Design review of the part built by this model. Coordinates are the model's own, in mm. A direction names the side the tool comes from. Coordinates: 2 decimals unless noted, no trailing zeros. Loops run counter-clockwise (first coordinate to the right, second up) from the corner with the lowest first, then second, coordinate; pieces in that order, holes last. Notation, with made-up numbers: (57.25, 68) -> (107.25, 68) arc R31 cw to (107.25, 100) -> close; hole circle Ø3 at (84.5, -39.5). An arc over 180 degrees is marked (long way). Answer in a Markdown table with one row per item.
Autodesk Fusion 360 part; units mm, degrees
sketch "Sketch1" plane through (0, 0, 0) normal (0, 0, 1) x (1, 0, 0)
  line L0 (0, 0) -> (50, 0)
  line L1 (50, 0) -> (50, 56)
  line L2 (50, 56) -> (0, 56)
  line L3 (0, 56) -> (0, 0)
  dimension "d1" = 50
  dimension "d2" = 56
extrude "Extrude1" add sketch "Sketch1" along normal blind 10
sketch "Sketch2" plane through (0, 0, 10) normal (0, 0, 1) x (-1, 0, 0)
  line L0 (0, -56) -> (0, 0)
  line L1 (0, 0) -> (-50, 0)
  line L2 (-50, 0) -> (-50, -56)
  line L3 (-50, -56) -> (0, -56)
  line L4 (0, 0) -> (-6, 0)
  line L5 (-6, 0) -> (-6, -6)
  circle A0 centre (-6, -6) radius 6
  line L6 (-50, 0) -> (-44, 0)
  line L7 (-44, 0) -> (-44, -6)
  circle A1 centre (-44, -6) radius 6
  dimension "d5" = 6
  dimension "d6" = 6
  dimension "d7" = 12
  dimension "d8" = 6
  dimension "d9" = 6
  dimension "d10" = 12
extrude "Extrude2" add sketch "Sketch2" along normal blind 2 contours A0 | A1
sketch "Sketch3" plane through (0, 0, 12) normal (0, 0, 1) x (-1, 0, 0)
  circle A0 centre (-6, -6) radius 6
  line L0 (-6, -6) -> (-12, -6)
sketch "Sketch4" plane through (0, 0, 12) normal (0, 0, 1) x (-1, 0, 0)
  circle A0 centre (-44, -6) radius 6
  line L0 (-44, -6) -> (-50, -6)
hole "Hole1" at (6, 6, 12) at (44, 6, 12) direction (0, 0, -1) diameter 5.035 depth 15 tip angle 118
sketch "Sketch5" plane through (0, 56, 0) normal (0, 1, 0) x (-1, 0, 0)
  line L0 (-50, 0) -> (0, 0)
  line L1 (0, 0) -> (0, 10)
  line L2 (0, 10) -> (-50, 10)
  line L3 (-50, 10) -> (-50, 0)
  line L4 (-50, 5) -> (-45, 5)
  line L5 (0, 5) -> (-5, 5)
  dimension "d23" = 5
  dimension "d24" = 5
hole "Hole3" at (45, 56, 5) at (5, 56, 5) direction (0, -1, 0) diameter 5.035 depth 18 tip angle 118
sketch "Sketch6" plane through (0, 56, 0) normal (0, 1, 0) x (-1, 0, 0)
  circle A0 centre (-45, 5) radius 2.5175
  circle A1 centre (-5, 5) radius 2.5175
  line L0 (-50, 0) -> (0, 0)
  line L1 (0, 0) -> (0, 10)
  line L2 (0, 10) -> (-50, 10)
  line L3 (-50, 10) -> (-50, 0)
  line L4 (-45, 5) -> (-35, 5)
  line L5 (-5, 5) -> (-15, 5)
  line L6 (-35, 5) -> (-35, 0)
  line L7 (-15, 5) -> (-15, 0)
  line L8 (-35, 0) -> (-38, 0)
  line L9 (-38, 0) -> (-38, 10)
  line L10 (-38, 10) -> (-35, 10)
  line L11 (-35, 10) -> (-35, 0)
  line L12 (-15, 0) -> (-12, 0)
  line L13 (-12, 0) -> (-12, 10)
  line L14 (-12, 10) -> (-15, 10)
  line L15 (-15, 10) -> (-15, 0)
  dimension "d28" = 10
  dimension "d29" = 10
  dimension "d30" = 3
  dimension "d31" = 3
extrude "Extrude3" add sketch "Sketch6" along normal blind 2 contours L2 L4 L9 L10 L11 | L0 L4 L6 L8 L9 L11 | L0 L5 L7 L12 L13 L15 | L2 L5 L13 L14 L15
sketch "Sketch7" plane through (0, 58, 0) normal (0, 1, 0) x (-1, 0, 0)
  line L0 (-35, 10) -> (-38, 10)
  line L1 (-38, 10) -> (-38, 0)
  line L2 (-38, 0) -> (-35, 0)
  line L3 (-35, 0) -> (-35, 10)
  line L4 (-35, 0) -> (-50, 0)
  line L5 (-50, 0) -> (-50, 10)
  line L6 (-50, 10) -> (-35, 10)
  line L7 (-35, 10) -> (-35, 0)
  line L8 (-35, 0) -> (0, 0)
  line L9 (0, 0) -> (0, 10)
  line L10 (0, 10) -> (-35, 10)
  line L11 (-35, 10) -> (-35, 0)
  dimension "d34" = 15
  dimension "d35" = 10
  dimension "d36" = 35
  dimension "d37" = 10
extrude "Extrude4" add sketch "Sketch7" along normal blind 8
sketch "Sketch8" plane through (0, 66, 0) normal (0, 1, 0) x (-1, 0, 0)
  line L0 (-50, 0) -> (0, 0)
  line L1 (0, 0) -> (0, 10)
  line L2 (0, 10) -> (-50, 10)
  line L3 (-50, 10) -> (-50, 0)
  line L4 (-50, 5) -> (-45, 5)
  line L5 (0, 5) -> (-5, 5)
  dimension "d40" = 5
  dimension "d41" = 5
hole "Hole4" at (45, 66, 5) at (5, 66, 5) direction (0, -1, 0) diameter 5.035 depth 28 tip angle 118
(1) Take a section at A-A on x = 25. Give the boundary of the cut face in (y, z), and give its area (3 significant figures).
Evaluation:
| item | result |
|---|---|
| outline | (0, 0) -> (56, 0) -> (56, 10) -> (0, 10) -> close; (58, 0) -> (66, 0) -> (66, 10) -> (58, 10) -> close |
| area | 640 mm² |
(2) Take a section at D-D on y = 7.5. Give the boundary of the cut face in (x, z).
Evaluation:
| item | result |
|---|---|
| outline | (0, 0) -> (3.98, 0) -> (3.98, 12) -> (0.19, 12) -> (0.19, 10) -> (0, 10) -> close; (8.02, 0) -> (41.98, 0) -> (41.98, 12) -> (38.19, 12) -> (38.19, 10) -> (11.81, 10) -> (11.81, 12) -> (8.02, 12) -> close; (46.02, 0) -> (50, 0) -> (50, 10) -> (49.81, 10) -> (49.81, 12) -> (46.02, 12) -> close |
(3) Take a section at B-B on y = 43. Give the boundary of the cut face in (x, z) (1 decimal).
Evaluation:
| item | result |
|---|---|
| outline | (0, 0) -> (50, 0) -> (50, 10) -> (0, 10) -> close; hole circle Ø5 at (5, 5); hole circle Ø5 at (45, 5) |
(4) Tool access review of faces 1 (the flat face through (35, 57, 5)), 2 (the flat face through (7.4, 58, 6.2)), 3 (the flat face through (49, 1, 10)), 4 (the flat face through (41, 58, 5)), 5 (the cylindrical face through (42.5, 61.9, 4.7)): name each direction out of +Z, -Z, +X, -X, +Y, -Y from which nothing blocks a thin tool from reaching the whole face with its end or side.
Evaluation:
| item | result |
|---|---|
| face 1 | +Z, -Z |
| face 2 | +Z, -Z, -X |
| face 3 | +Z, +X, -Y |
| face 4 | +Z, -Z, +X |
| face 5 | +Y |
(5) To check wall thickness, follow probe 1 along Y at (x, z) = (44, 7.5); probe 2 along X at (y, z) = (6, 5); probe 3 along X at (y, z) = (62.5, 5). State the ranges of each line that lie inside material, in increasing order.
Evaluation:
| item | result |
|---|---|
| probe 1 | y = 0 to 3.48, 8.52 to 56, 58 to 66 |
| probe 2 | x = 0 to 3.48, 8.52 to 41.48, 46.52 to 50 |
| probe 3 | x = 0 to 2.48, 7.52 to 42.48, 47.52 to 50 |
(6) Take a section at C-C on z = 6.75. Count the separate pieces of the cut face and the enclosed holes in it, and give its area (3 significant figures).
Evaluation:
| item | result |
|---|---|
| separate pieces | 3 |
| enclosed holes | 3 |
| area | 2,980 mm² |
(7) For pin 1 (3 mm diameter, centred on x = 5, z = 5, fed in from +Y); pin 2 (2 mm diameter, centred on x = 8.5, y = 49, fed in from +Z), all flat-tipped, find the tip position at first contact; note any pin that passes through.
Evaluation:
| item | result |
|---|---|
| pin 1 | stops at y = 37.39 |
| pin 2 | stops at z = 10 |
(8) Draft analysis for pull direction X (two halves, no side actions). For faces 6 (the conical face through (45.43, 36.75, 4.94)), 7 (the flat face through (41, 6, 12)), 8 (the flat face through (50, 28, 5)), state which applies: pulls with the +X half, pulls with the -X half, needs draft (parallel to the pull), parting line crosses it, or undercut.
Evaluation:
| item | result |
|---|---|
| face 6 | undercut |
| face 7 | needs draft |
| face 8 | pulls with the +X half |
